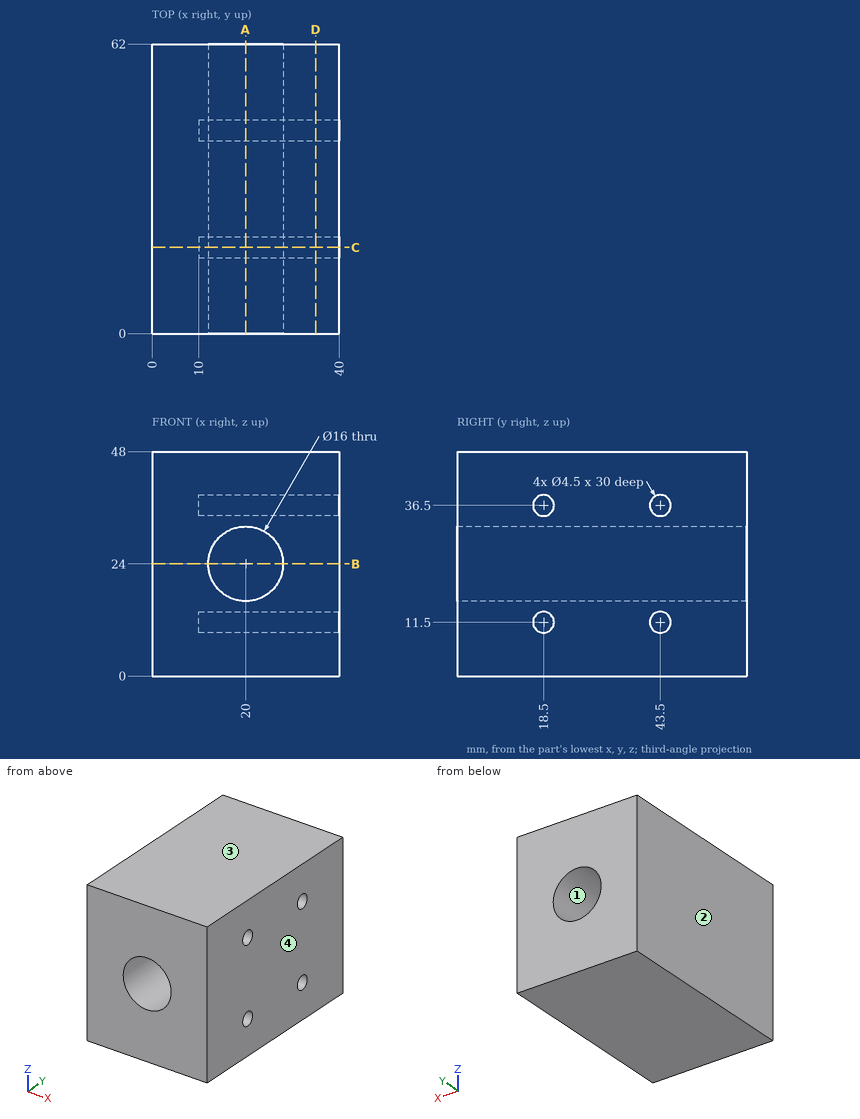
Design review of the part shown in the three views and the two pictorial views. Dimensions are in mm from the part's minimum x, y and z. Round coordinates to 2 decimals unless told otherwise and drop trailing zeros. Write each loop counter-clockwise with the first axis right and the second up, starting at its lowest first coordinate (ties: lowest second). Pieces come first, ordered by that corner, then holes. Notation, with made-up numbers: (41, -4.75) - (98, -4.75) arc R30 ccw to (98, 30.25) - close; hole circle Ø6 at (69.5, 26.25). An arc over 180 degrees is marked (long way). Write item = value, one per line. Start each with the question number.
1. Consider section C-C on y = 18.5. State the section outline as (x, z) points.
2. Consider section B-B on z = 24. State the section outline as (x, y) points, plus the area to 3 significant figures.
3. Wall thickness on L1, parallel to Y at x = 19.75, z = 11.5; L2, parallel to Z at x = 27, y = 43; L3, parallel to Z at x = 19.5, y = 25.5: over which ranges is each line inside the solid? List them lowest first.
4. Consider section D-D on x = 35. State the section outline as (y, z) points.
5. Draft analysis for pull direction X (two halves, no side actions). For the marked faces 1, 2, 3 and 4, state which applies: released by +X, released by -X, zero draft, split by the parting line, or undercut.
6. Consider section A-A on x = 20. State the section outline as (y, z) points.
7. For pin 1 Ø5 at (y, z) = (18.5, 12) entering from +X; pin 2 Ø2 at (y, z) = (44.5, 11) entering from +X, all flat-tipped, find the tip position at first contact; note any pin that passes through.
Evaluation:
q1.outline = (0, 0) - (40, 0) - (40, 9.25) - (10, 9.25) - (10, 13.75) - (40, 13.75) - (40, 34.25) - (10, 34.25) - (10, 38.75) - (40, 38.75) - (40, 48) - (0, 48) - close; hole circle Ø16 at (20, 24)
q2.outline = (0, 0) - (12, 0) - (12, 62) - (0, 62) - close; (28, 0) - (40, 0) - (40, 62) - (28, 62) - close
q2.area = 1,490 mm2
q3.L1 = 0 to 16.25, 20.75 to 41.25, 45.75 to 62
q3.L2 = 0 to 9.31, 13.69 to 20.13, 27.87 to 34.31, 38.69 to 48
q3.L3 = 0 to 16.02, 31.98 to 48
q4.outline = (0, 0) - (62, 0) - (62, 48) - (0, 48) - close; hole circle Ø4.5 at (18.5, 11.5); hole circle Ø4.5 at (18.5, 36.5); hole circle Ø4.5 at (43.5, 11.5); hole circle Ø4.5 at (43.5, 36.5)
q5.face_1 = undercut
q5.face_2 = released by -X
q5.face_3 = zero draft
q5.face_4 = released by +X
q6.outline = (0, 0) - (62, 0) - (62, 16) - (0, 16) - close; (0, 32) - (62, 32) - (62, 48) - (0, 48) - close; hole circle Ø4.5 at (18.5, 11.5); hole circle Ø4.5 at (18.5, 36.5); hole circle Ø4.5 at (43.5, 11.5); hole circle Ø4.5 at (43.5, 36.5)
q7.pin_1 = 40
q7.pin_2 = 10
